Part model, mm, in its own coordinate system. A direction names the side the tool comes from. Round coordinates to 2 decimals unless told otherwise and drop trailing zeros. Loops run counter-clockwise (first coordinate to the right, second up) from the corner with the lowest first, then second, coordinate; pieces in that order, holes last.
(1) Flat gauge pins, fed straight in: pin 1 (1.2 mm diameter, centred on x = 6, z = 21, fed in from +Y); pin 2 (1.5 mm diameter, centred on y = 5, z = 7.5, fed in from -X); pin 3 (3 mm diameter, centred on x = -5, z = 17.5, fed in from -Y); pin 4 (10 mm diameter, centred on y = 6, z = 31, fed in from -X). Where does each tip first touch, or does it go through?
(2) Cut at B-B on y = -5. List the corners of the cut face in (x, z).
(3) Tool access for faces 1 (the face through (-6, -2.5, 17)), 2 (the face through (6, 2.5, 17)), 3 (the face through (-2.5, 6, 17)), 4 (the face through (2.5, -6, 17)): list every direction of +Z, -Z, +X, -X, +Y, -Y with a clear straight run to the whole face (end or side of a thin tool).
(4) Probe probe 1 along X at (y, z) = (5.25, 28); probe 2 along Y at (x, z) = (-8, 32.5). List the from-to ranges inside material, lowest first.
(5) Cut at A-A on z = 10. List the corners of the cut face in (x, y).
from build123d import *

# Parameters (mm, degrees)
F1_DEPTH = 35
F2_R     = 1
F3_R     = 1
F4_R     = 1


with BuildPart() as f1:
    # F0 (on Top) → F1 (new body)
    with BuildSketch(Plane.XY):
        Polygon((-8.5, -2.5), (-2.5, -2.5), (-2.5, -8.5), (2.5, -8.5), (2.5, -2.5), (8.5, -2.5), (8.5, 2.5), (2.5, 2.5), (2.5, 8.5), (-2.5, 8.5), (-2.5, 2.5), (-8.5, 2.5), align=None)
    extrude(amount=F1_DEPTH)

    # F2
    f2_edges = [f1.edges().sort_by_distance(p)[0] for p in [
        (2.5, -2.5, 17.5),
        (-2.5, -2.5, 17.5),
    ]]
    fillet(f2_edges, radius=F2_R)

    # F3
    f3_edges = [f1.edges().sort_by_distance(p)[0] for p in [
        (-2.5, 2.5, 17.5),
        (2.5, 2.5, 17.5),
    ]]
    fillet(f3_edges, radius=F3_R)

    # F4
    f4_edges = [f1.edges().sort_by_distance(p)[0] for p in [
        (-2.5, -8.5, 17.5),
        (2.5, -8.5, 17.5),
        (-8.5, -2.5, 17.5),
        (-8.5, 2.5, 17.5),
        (-2.5, 8.5, 17.5),
        (2.5, 8.5, 17.5),
        (8.5, 2.5, 17.5),
        (8.5, -2.5, 17.5),
    ]]
    fillet(f4_edges, radius=F4_R)


solid = f1.part
Final values:
1. pin 1: stops at y = 2.5
1. pin 2: stops at x = -2.5
1. pin 3: stops at y = -2.5
1. pin 4: stops at x = -8.5
2. outline: (-2.5, 0) - (2.5, 0) - (2.5, 35) - (-2.5, 35) - close
3. face 1: +Z, -Z, -X, -Y
3. face 2: +Z, -Z, +X, +Y
3. face 3: +Z, -Z, -X, +Y
3. face 4: +Z, -Z, +X, -Y
4. probe 1: x = -2.5 to 2.5
4. probe 2: y = -2.37 to 2.37
5. outline: (-8.5, -1.5) arc R1 ccw to (-7.5, -2.5) - (-3.5, -2.5) arc R1 cw to (-2.5, -3.5) - (-2.5, -7.5) arc R1 ccw to (-1.5, -8.5) - (1.5, -8.5) arc R1 ccw to (2.5, -7.5) - (2.5, -3.5) arc R1 cw to (3.5, -2.5) - (7.5, -2.5) arc R1 ccw to (8.5, -1.5) - (8.5, 1.5) arc R1 ccw to (7.5, 2.5) - (3.5, 2.5) arc R1 cw to (2.5, 3.5) - (2.5, 7.5) arc R1 ccw to (1.5, 8.5) - (-1.5, 8.5) arc R1 ccw to (-2.5, 7.5) - (-2.5, 3.5) arc R1 cw to (-3.5, 2.5) - (-7.5, 2.5) arc R1 ccw to (-8.5, 1.5) - close
